Build history of the part. All positions in model axes, mm. Round coordinates to 2 decimals unless told otherwise and drop trailing zeros. Write each loop counter-clockwise with the first axis right and the second up, starting at its lowest first coordinate (ties: lowest second). Pieces come first, ordered by that corner, then holes. Notation, with made-up numbers: M 70,42 L 92,42 A22 cw 92,48 Z; hole C 86,79 d3. An arc over 180 degrees is marked long. Use a Markdown table: item, result.
from build123d import *

# Parameters (mm, degrees)
EXTRUDE_3_DEPTH     = 5
SKETCH_12_W         = 25
SKETCH_12_H         = 25
CUT_EXTRUDE_2_DEPTH = 5
CUT_EXTRUDE_3_DEPTH = 5
SKETCH_14_R         = 4.1
CUT_EXTRUDE_4_DEPTH = 5
SKETCH_16_R         = 3.1
CUT_EXTRUDE_5_DEPTH = 5
CUT_EXTRUDE_6_DEPTH = 5
SKETCH_18_W         = 25
SKETCH_18_H         = 35
EXTRUDE_4_DEPTH     = 5
CUT_EXTRUDE_7_DEPTH = 5


with BuildPart() as part:
    # 草图8 → 凸台-拉伸3 (new body)
    with BuildSketch(Plane.XY):
        with BuildLine():
            Line((-12.5, 150), (12.5, 150))
            Line((12.5, 150), (12.5, 27.271780287))
            ThreePointArc((12.5, 27.271780287), (0, -30), (-12.5, 27.271780287))
            Line((-12.5, 27.271780287), (-12.5, 150))
        make_face()
    extrude(amount=EXTRUDE_3_DEPTH)

    # 草图12 → 切除-拉伸2 (cut)
    with BuildSketch(Plane.XY.offset(5)):
        with Locations((0, 137.5)):
            Rectangle(SKETCH_12_W, SKETCH_12_H)
    extrude(amount=-CUT_EXTRUDE_2_DEPTH, mode=Mode.SUBTRACT)

    # 草图13 → 切除-拉伸3 (cut)
    with BuildSketch(Plane.XY.offset(5)):
        Polygon((-12.5, 125), (12.5, 125), (-12.5, 100), align=None)
    extrude(amount=-CUT_EXTRUDE_3_DEPTH, mode=Mode.SUBTRACT)

    # 草图14 → 切除-拉伸4 (cut)
    with BuildSketch(Plane.XY.offset(5)):
        Circle(SKETCH_14_R)
    extrude(amount=-CUT_EXTRUDE_4_DEPTH, mode=Mode.SUBTRACT)

    # 草图16 → 切除-拉伸5 (cut)
    with BuildSketch(Plane.XY.offset(5)):
        with Locations((0, -25)):
            Circle(SKETCH_16_R)
        with Locations((-9.031041655, -23.311805735)):
            Circle(SKETCH_16_R)
        with Locations((-16.842391091, -18.475222931)):
            Circle(SKETCH_16_R)
        with Locations((-22.379082284, -11.143458894)):
            Circle(SKETCH_16_R)
        with Locations((-24.893354407, -2.306708987)):
            Circle(SKETCH_16_R)
        with Locations((-24.045641079, 6.841574752)):
            Circle(SKETCH_16_R)
        with Locations((-19.950430682, 15.065865909)):
            Circle(SKETCH_16_R)
        with Locations((-13.160804072, 21.255428393)):
            Circle(SKETCH_16_R)
        with Locations((-4.593737945, 24.574327492)):
            Circle(SKETCH_16_R)
        with Locations((4.593737945, 24.574327492)):
            Circle(SKETCH_16_R)
        with Locations((13.160804072, 21.255428393)):
            Circle(SKETCH_16_R)
        with Locations((19.950430682, 15.065865909)):
            Circle(SKETCH_16_R)
        with Locations((24.045641079, 6.841574752)):
            Circle(SKETCH_16_R)
        with Locations((24.893354407, -2.306708987)):
            Circle(SKETCH_16_R)
        with Locations((22.379082284, -11.143458894)):
            Circle(SKETCH_16_R)
        with Locations((16.842391091, -18.475222931)):
            Circle(SKETCH_16_R)
        with Locations((9.031041655, -23.311805735)):
            Circle(SKETCH_16_R)
    extrude(amount=-CUT_EXTRUDE_5_DEPTH, mode=Mode.SUBTRACT)

    # 草图17 → 切除-拉伸6 (cut)
    with BuildSketch(Plane.XY.offset(5)):
        Polygon((-12.5, 100), (12.5, 125), (12.5, 95), (-12.5, 70), align=None)
    extrude(amount=-CUT_EXTRUDE_6_DEPTH, mode=Mode.SUBTRACT)

    # 草图18 → 凸台-拉伸4 (add)
    with BuildSketch(Plane.XY.offset(5)):
        with Locations((0, 87.5)):
            Rectangle(SKETCH_18_W, SKETCH_18_H)
    extrude(amount=-EXTRUDE_4_DEPTH)

    # 草图19 → 切除-拉伸7 (cut)
    with BuildSketch(Plane.XY.offset(5)):
        Polygon((-12.5, 105), (12.5, 105), (-12.5, 80), align=None)
    extrude(amount=-CUT_EXTRUDE_7_DEPTH, mode=Mode.SUBTRACT)


solid = part.part
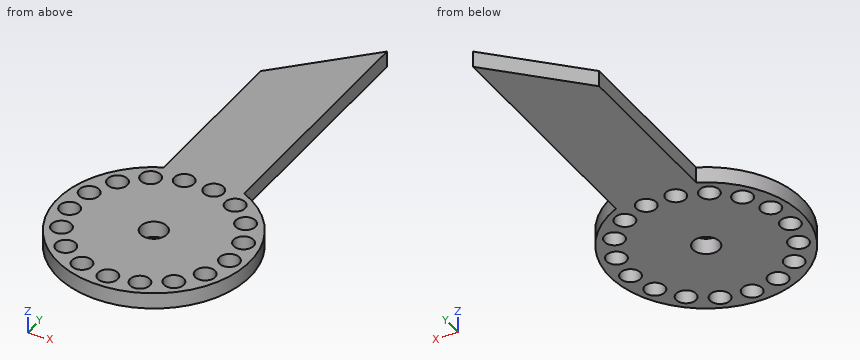
Q1. Cut at D-D on y = 55.5. Give the cut face in (x, z), and give its area (3 significant figures).
Response values:
| item | result |
|---|---|
| outline | M -12.5,0 L 12.5,0 L 12.5,5 L -12.5,5 Z |
| area | 125 mm2 |
Q2. Cut at B-B on y = -25. Give the cut face in (x, z), and give its area (3 significant figures).
Response values:
| item | result |
|---|---|
| outline | M -16.58,0 L -11.63,0 L -11.63,5 L -16.58,5 Z; M -6.43,0 L -3.1,0 L -3.1,5 L -6.43,5 Z; M 3.1,0 L 6.43,0 L 6.43,5 L 3.1,5 Z; M 11.63,0 L 16.58,0 L 16.58,5 L 11.63,5 Z |
| area | 82.8 mm2 |
Q3. Drop flat-ended pins along their axis: P1, Ø8, axis at x = 24.05, y = 6.84, coming from the +Z side; P2, Ø2, axis at y = 46.5, z = 3, coming from the +X side; P3, Ø3, axis at x = 2, z = 1.5, coming from the +Y side; P4, Ø5.5, axis at x = -24.05, y = 6.84, coming from the -Z side. Give the stop position or say it passes through.
Response values:
| item | result |
|---|---|
| P1 | stops at z = 5 |
| P2 | stops at x = 12.5 |
| P3 | stops at y = 96 |
| P4 | passes through |
Q4. Cut at C-C on z = 3. Count the separate pieces of the cut face and the enclosed holes in it, and give its area (3 significant figures).
Response values:
| item | result |
|---|---|
| separate pieces | 1 |
| enclosed holes | 18 |
| area | 3,850 mm2 |
Q5. Drill centre lines: L1, parallel to Y at x = -14, z = 4.15; L2, parallel to X at y = 20, z = 1.45; L3, parallel to Y at x = 25, z = 4.5. Where is each one in solid material? Low to high.
Response values:
| item | result |
|---|---|
| L1 | y = -26.53 to -19.71, -17.24 to 18.27, 24.24 to 26.53 |
| L2 | x = -22.36 to -16, -10.33 to 10.33, 16 to 22.36 |
| L3 | y = -16.58 to -12.8, -9.49 to -5.4, 0.79 to 3.89, 9.79 to 16.58 |
Q6. Cut at A-A on x = 0. Give the cut face in (y, z).
Response values:
| item | result |
|---|---|
| outline | M -30,0 L -28.1,0 L -28.1,5 L -30,5 Z; M -21.9,0 L -4.1,0 L -4.1,5 L -21.9,5 Z; M 4.1,0 L 92.5,0 L 92.5,5 L 4.1,5 Z |
